```python
from build123d import *

# Parameters (mm, degrees)
SKETCH1_R               = 30
SKETCH1_R_2             = 15
BOSS_EXTRUDE1_DEPTH     = 80
SKETCH2_W               = 30
SKETCH2_H               = 60
CUT_EXTRUDE1_DEPTH      = 40
CUT_EXTRUDE2_DEPTH      = 97.566039579
CUT_EXTRUDE2_DEPTH_BACK = 97.566039579
SKETCH3_R               = 5
BOSS_EXTRUDE2_START     = -10
SKETCH4_R               = 15
BOSS_EXTRUDE2_DEPTH     = 10
CUT_EXTRUDE3_DEPTH      = 91.553851536
CUT_EXTRUDE3_DEPTH_BACK = 91.553851536
SKETCH5_R               = 5


with BuildPart() as part:
    # Sketch1 → Boss-Extrude1 (new body)
    with BuildSketch(Plane(origin=(0, 0, 0), x_dir=(1, 0, 0), z_dir=(0, 1, 0))):
        with Locations(Location((0, 0, 0), (0, 0, 270))):
            Circle(SKETCH1_R)
        with Locations(Location((0, 0, 0), (0, 0, 270))):
            Circle(SKETCH1_R_2, mode=Mode.SUBTRACT)
    extrude(amount=BOSS_EXTRUDE1_DEPTH)

    # Sketch2 → Cut-Extrude1 (cut)
    with BuildSketch(Plane(origin=(0, 80, 0), x_dir=(1, 0, 0), z_dir=(0, 1, 0))):
        Rectangle(SKETCH2_W, SKETCH2_H)
    extrude(amount=-CUT_EXTRUDE1_DEPTH, mode=Mode.SUBTRACT)

    # Sketch3 → Cut-Extrude2 (cut, two sides: drawn at the far end of the back side and taken through both)
    with BuildSketch(Plane(origin=(-15, 0, 0), x_dir=(0, 0, -1), z_dir=(1, 0, 0)).offset(-CUT_EXTRUDE2_DEPTH_BACK)):
        with Locations(Location((0, 70, 0), (0, 0, 270))):
            Circle(SKETCH3_R)
    extrude(amount=CUT_EXTRUDE2_DEPTH + CUT_EXTRUDE2_DEPTH_BACK, mode=Mode.SUBTRACT)

    # Sketch4 → Boss-Extrude2 (add)
    with BuildSketch(Plane(origin=(0, 40, 0), x_dir=(1, 0, 0), z_dir=(0, 1, 0)).offset(BOSS_EXTRUDE2_START)):
        with Locations(Location((0, 0, 0), (0, 0, 270))):
            Circle(SKETCH4_R)
    extrude(amount=BOSS_EXTRUDE2_DEPTH)

    # Sketch5 → Cut-Extrude3 (cut, two sides: drawn at the far end of the back side and taken through both)
    with BuildSketch(Plane(origin=(0, 0, 0), x_dir=(0, 0, -1), z_dir=(1, 0, 0)).offset(-CUT_EXTRUDE3_DEPTH_BACK)):
        with Locations((0, 10)):
            Circle(SKETCH5_R)
    extrude(amount=CUT_EXTRUDE3_DEPTH + CUT_EXTRUDE3_DEPTH_BACK, mode=Mode.SUBTRACT)


solid = part.part
```
Geometry: final body of the model. Coordinates: model frame, mm. A direction names the side the tool comes from. Round coordinates to 2 decimals unless told otherwise and drop trailing zeros. Order: outer loops, then holes, each group sorted by start corner. A loop starts at its lowest first (then second) coordinate and runs counter-clockwise, first axis right, second up. Notation, with made-up numbers: (89, -5) - (106, -5) arc R35 ccw to (106, 32) - close; hole circle Ø7 at (40, 14.25). An arc over 180 degrees is marked (long way). Write item = value, one per line. Start each with the question number.
Q1. Pull-direction query (Z, two-part tool) for faces 1 (the flat face through (-21, 80, 0)), 2 (the cylindrical face through (1.32, 39.44, -29.97)), 3 (the cylindrical face through (22.395, 65.381, 1.915)); classes: +Z half, -Z half, draft (parallel to the pull), parting line (faces both ways), or undercut.
Q2. Cut plane B-B on y = 70. Return the cut outline in (x, z).
Q3. Cut plane D-D on y = 10. Return the cut outline in (x, z).
Q4. Access query for faces 4 (the cylindrical face through (-22.605, 65.381, 1.915)), 5 (the flat face through (-15, 60, 0)), 6 (the flat face through (0, 30, 0)). Directions: +Z, -Z, +X, -X, +Y, -Y. A direction counts if a zero-diameter tool reaches every point of the face in a straight line with its end or side. Return the directions, or none.
Q5. Cut plane A-A on z = 0. Return the cut outline in (x, y).
Q6. Cut plane C-C on x = 0. Return the cut outline in (y, z), and give its area (3 significant figures).
Q7. Pin query (flat end, axial travel): pin 1 (12 mm diameter, centred on x = 15, y = 31, fed in from +Z); pin 2 (1.5 mm diameter, centred on x = 3.5, y = 38.5, fed in from -Z); pin 3 (2 mm diameter, centred on y = 36, z = -22.5, fed in from -X); pin 4 (9 mm diameter, centred on y = 70, z = 0, fed in from +X). Return the tip coordinate at first contact, or that it passes through.
Q8. Ray query, line 1 (X direction, y = 17.5, z = 0); line 2 (Z direction, x = 0.5, y = 9); line 3 (Y direction, x = -25, z = 1.5). Return the intervals inside material, ascending. Write a range as from..to.
Outcome:
q1.face_1 = draft
q1.face_2 = parting line
q1.face_3 = undercut
q2.outline = (-29.58, -5) arc R30 ccw to (-15, -25.98) - (-15, -5) - close; (-29.58, 5) - (-15, 5) - (-15, 25.98) arc R30 ccw to start; (15, -25.98) arc R30 ccw to (29.58, -5) - (15, -5) - close; (15, 5) - (29.58, 5) arc R30 ccw to (15, 25.98) - close
q3.outline = (-29.58, -5) arc R30 ccw to (29.58, -5) - (14.14, -5) arc R15 cw to (-14.14, -5) - close; (-29.58, 5) - (-14.14, 5) arc R15 cw to (14.14, 5) - (29.58, 5) arc R30 ccw to start
q4.face_4 = +X, -X
q4.face_5 = +Z, -Z, +Y
q4.face_6 = -Y
q5.outline = (-30, 0) - (-15, 0) - (-15, 5) - (-30, 5) - close; (-30, 15) - (-15, 15) - (-15, 30) - (15, 30) - (15, 15) - (30, 15) - (30, 65) - (15, 65) - (15, 40) - (-15, 40) - (-15, 65) - (-30, 65) - close; (-30, 75) - (-15, 75) - (-15, 80) - (-30, 80) - close; (15, 0) - (30, 0) - (30, 5) - (15, 5) - close; (15, 75) - (30, 75) - (30, 80) - (15, 80) - close
q6.outline = (0, -30) - (40, -30) - (40, 30) - (0, 30) - (0, 15) - (30, 15) - (30, -15) - (0, -15) - close
q6.area = 1,500 mm^2
q7.pin_1 = 28.62
q7.pin_2 = -29.87
q7.pin_3 = -20.92
q7.pin_4 = through
q8.line_1 = -30..-15, 15..30
q8.line_2 = -30..-14.99, 14.99..30
q8.line_3 = 0..5.23, 14.77..65.23, 74.77..80
